```python
from build123d import *

# Parameters (mm, degrees)
SKETCH1_W                       = 254
SKETCH1_H                       = 6.35
BASE_EXTRUSION_DEPTH            = 94.968888282
SKETCH4_W                       = 25.4
SKETCH4_H                       = 6.35
TAB_HOLES_TO_CHASSIS_BASE_DEPTH = 173.608322449
T_SLOT_CENTER_DEPTH             = 173.608322449
SKETCH6_W                       = 31.75
SKETCH6_H                       = 104.14
ARM_SUPPORT_DEPTH               = 6.35
SKETCH8_W                       = 12.7
SKETCH8_H                       = 6.35
ARM_CLEARANCE_DEPTH             = 90.206388282
SKETCH9_R                       = 2.0955
BASE_MOUNTING_HOLE_1_DEPTH      = 246.802548054
SKETCH10_R                      = 2.0955
BASE_MOUNTING_HOLE_2_DEPTH      = 246.802548054
SKETCH11_R                      = 2.0955
ARM_SUPPORT_MOUNTING_HOLE_DEPTH = 246.802548054
SKETCH12_W                      = 6.35
SKETCH12_H                      = 12.7
ARM_SUPPORT_TAB_SLOTS_DEPTH     = 246.802548054
T_START                         = -6.35
T_SLOT_TOP_CORNER_DEPTH         = 6.35
T_SLOT_TOP_CORNER_2_OUTLINE_W   = 25.4
T_SLOT_TOP_CORNER_2_OUTLINE_H   = 6.35
T_SLOT_TOP_CORNER_2_OUTLINE_W_2 = 16.5312
T_SLOT_TOP_CORNER_2_DEPTH       = 6.35
SKETCH15_R                      = 2.0955
CUT_EXTRUDE8_DEPTH              = 246.802548054


# Read off the part's stored shape, not the designer's step: T Slot Top Corner
with BuildPart() as part:
    # Sketch1 → Base Extrusion (new body)
    with BuildSketch(Plane(origin=(0, 0, 0), x_dir=(1, 0, 0), z_dir=(0, 1, 0))):
        with Locations((-16.993821871, 0)):
            Rectangle(SKETCH1_W, SKETCH1_H)
    extrude(amount=BASE_EXTRUSION_DEPTH)

    # Sketch4 → Tab Holes to Chassis Base (cut, through all)
    with BuildSketch(Plane.XY.offset(3.175)):
        with Locations((-55.093821871, 9.243888282)):
            Rectangle(SKETCH4_W, SKETCH4_H)
        with Locations((-16.993821871, 9.243888282)):
            Rectangle(SKETCH4_W, SKETCH4_H)
        with Locations((21.106178129, 9.243888282)):
            Rectangle(SKETCH4_W, SKETCH4_H)
    extrude(amount=-TAB_HOLES_TO_CHASSIS_BASE_DEPTH, mode=Mode.SUBTRACT)

    # Sketch5 → T Slot Center (cut, through all)
    with BuildSketch(Plane.XY.offset(3.175)):
        Polygon((-14.860221871, 94.968888282), (-19.127421871, 94.968888282), (-19.127421871, 86.205888282), (-21.438821871, 86.205888282), (-21.438821871, 83.030888282), (-19.127421871, 83.030888282), (-19.127421871, 79.728888282), (-14.860221871, 79.728888282), (-14.860221871, 83.030888282), (-12.548821871, 83.030888282), (-12.548821871, 86.205888282), (-14.860221871, 86.205888282), align=None)
    extrude(amount=-T_SLOT_CENTER_DEPTH, mode=Mode.SUBTRACT)

    # Sketch6 → Arm Support (add)
    with BuildSketch(Plane.XY.offset(3.175)):
        with Locations((46.506178129, 147.038888282)):
            Rectangle(SKETCH6_W, SKETCH6_H)
    extrude(amount=-ARM_SUPPORT_DEPTH)

    # Sketch8 → Arm Clearance (cut)
    with BuildSketch(Plane(origin=(0, 94.968888282, 0), x_dir=(1, 0, 0), z_dir=(0, 1, 0))):
        with Locations((87.124978129, 0)):
            Rectangle(SKETCH8_W, SKETCH8_H)
    extrude(amount=-ARM_CLEARANCE_DEPTH, mode=Mode.SUBTRACT)

    # Sketch9 → Base Mounting Hole 1 (cut, through all)
    with BuildSketch(Plane.XY.offset(3.175)):
        with Locations((101.740578129, 9.243888282)):
            Circle(SKETCH9_R)
    extrude(amount=-BASE_MOUNTING_HOLE_1_DEPTH, mode=Mode.SUBTRACT)

    # Sketch10 → Base Mounting Hole 2 (cut, through all)
    with BuildSketch(Plane.XY.offset(3.175)):
        with Locations((-105.893821871, 9.243888282)):
            Circle(SKETCH10_R)
    extrude(amount=-BASE_MOUNTING_HOLE_2_DEPTH, mode=Mode.SUBTRACT)

    # Sketch11 → Arm Support Mounting Hole (cut, through all)
    with BuildSketch(Plane.XY.offset(3.175)):
        with Locations((59.206178129, 147.038888282)):
            Circle(SKETCH11_R)
    extrude(amount=-ARM_SUPPORT_MOUNTING_HOLE_DEPTH, mode=Mode.SUBTRACT)

    # Sketch12 → Arm Support Tab Slots (cut, through all)
    with BuildSketch(Plane.XY.offset(3.175)):
        with Locations((59.206178129, 172.438888282)):
            Rectangle(SKETCH12_W, SKETCH12_H)
        with Locations((59.206178129, 121.638888282)):
            Rectangle(SKETCH12_W, SKETCH12_H)
    extrude(amount=-ARM_SUPPORT_TAB_SLOTS_DEPTH, mode=Mode.SUBTRACT)

    # T Slot Top Corner outline → T Slot Top Corner (cut)
    with BuildSketch(Plane.XY.offset(3.175).offset(T_START)):
        Polygon((-126.848821871, 83.030888282), (-126.848821871, 86.205888282), (-129.160221871, 86.205888282), (-129.160221871, 94.968888282), (-133.427421871, 94.968888282), (-133.427421871, 86.205888282), (-135.738821871, 86.205888282), (-135.738821871, 83.030888282), (-133.427421871, 83.030888282), (-133.427421871, 79.728888282), (-129.160221871, 79.728888282), (-129.160221871, 83.030888282), align=None)
    extrude(amount=T_SLOT_TOP_CORNER_DEPTH, mode=Mode.SUBTRACT)

    # T Slot Top Corner 2 outline → T Slot Top Corner 2 (add)
    with BuildSketch(Plane.XY.offset(3.175).offset(T_START)):
        with Locations((-62.510621871, 98.143888282)):
            Rectangle(T_SLOT_TOP_CORNER_2_OUTLINE_W, T_SLOT_TOP_CORNER_2_OUTLINE_H)
        with Locations((-105.893821871, 98.143888282)):
            Rectangle(T_SLOT_TOP_CORNER_2_OUTLINE_W, T_SLOT_TOP_CORNER_2_OUTLINE_H)
        with Locations((101.740578129, 98.143888282)):
            Rectangle(T_SLOT_TOP_CORNER_2_OUTLINE_W_2, T_SLOT_TOP_CORNER_2_OUTLINE_H)
        with Locations((7.885478129, 98.143888282)):
            Rectangle(T_SLOT_TOP_CORNER_2_OUTLINE_W, T_SLOT_TOP_CORNER_2_OUTLINE_H)
    extrude(amount=T_SLOT_TOP_CORNER_2_DEPTH)

    # Sketch15 → Cut-Extrude8 (cut, through all)
    with BuildSketch(Plane.XY.offset(3.175)):
        with Locations((101.740578129, 98.143888282)):
            Circle(SKETCH15_R)
    extrude(amount=-CUT_EXTRUDE8_DEPTH, mode=Mode.SUBTRACT)


solid = part.part
```
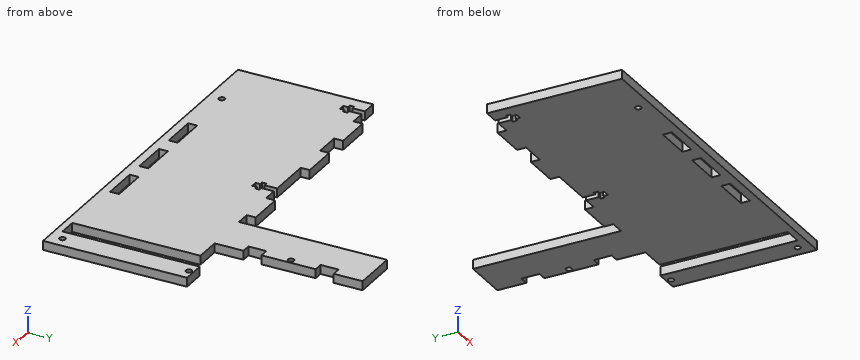
Design review of the part built by this model. Coordinates are the model's own, in mm. Give positions to 0.01 mm unless a question says otherwise; leave off trailing zeros. Order: outer loops, then holes, each group sorted by start corner. A loop starts at its lowest first (then second) coordinate and runs counter-clockwise, first axis right, second up. Notation, with made-up numbers: (1, -3) -> (11, -3) arc R13 ccw to (11, 10) -> close; hole circle Ø5 at (31.5, 40.5). An arc over 180 degrees is marked (long way). Write each question's results on one line, items separated by ' | '. Start each with the question number.
Q1. Add section C-C on y = 91.5. Give the boundary of the cut face in (x, z) (3 decimals), and give its area (3 significant figures).
Q2. For pin 1 (1 mm diameter, centred on x = -9.5, z = 0.5, fed in from +Y), flat-tipped, find the tip position at first contact; note if it passes through.
Q3. Wall thickness on L1, parallel to X at y = 80, z = -1.5; L2, parallel to X at y = 76, z = 0; L3, parallel to Y at x = 24, z = 1.5: over which ranges is each line inside the solid? List them lowest first. Write a range as from..to.
Q4. Add section B-B on x = 13. Give the boundary of the cut face in (y, z) (3 decimals), and give its area (3 significant figures).
Q5. Add section A-A on y = 29. Give the boundary of the cut face in (x, z) (3 decimals).
Q6. Add section D-D on x = -114.5. Give the boundary of the cut face in (y, z) (3 decimals).
Found:
1) outline: (-143.994, -3.175) -> (-133.427, -3.175) -> (-133.427, 3.175) -> (-143.994, 3.175) -> close; (-129.16, -3.175) -> (-19.127, -3.175) -> (-19.127, 3.175) -> (-129.16, 3.175) -> close; (-14.86, -3.175) -> (80.775, -3.175) -> (80.775, 3.175) -> (-14.86, 3.175) -> close; (93.475, -3.175) -> (110.006, -3.175) -> (110.006, 3.175) -> (93.475, 3.175) -> close | area: 1,480 mm2
2) pin 1: stops at y = 94.97
3) L1: x = -143.99..-133.43, -129.16..-19.13, -14.86..80.77, 93.47..110.01 | L2: x = -143.99..80.77, 93.47..110.01 | L3: y = 0..6.07, 12.42..94.97
4) outline: (0, -3.175) -> (6.069, -3.175) -> (6.069, 3.175) -> (0, 3.175) -> close; (12.419, -3.175) -> (101.319, -3.175) -> (101.319, 3.175) -> (12.419, 3.175) -> close | area: 603 mm2
5) outline: (-143.994, -3.175) -> (80.775, -3.175) -> (80.775, 3.175) -> (-143.994, 3.175) -> close; (93.475, -3.175) -> (110.006, -3.175) -> (110.006, 3.175) -> (93.475, 3.175) -> close
6) outline: (0, -3.175) -> (101.319, -3.175) -> (101.319, 3.175) -> (0, 3.175) -> close
